CAD build for the part. Positions are in the model's coordinates, mm. A direction names the side the tool comes from. Give positions to 0.01 mm unless a question says otherwise; leave off trailing zeros. Write each loop counter-clockwise with the first axis right and the second up, starting at its lowest first coordinate (ties: lowest second). Pieces come first, ordered by that corner, then holes. Notation, with made-up numbers: M -36.75,-2.75 L 18.25,-2.75 A18 cw 18.25,19.25 Z; hole C 0,-1.5 d5. An arc over 180 degrees is marked long. One line per question, with ' | ' between items. Start each with the question number.
1. Pull direction X, two halves, no side cores. Call faces 1 (the face through (3.2, -3.2, 5.5)), 2 (the face through (1.75, 5, 3)), 3 (the face through (-7.493, 0.33, 2.712)), 4 (the face through (0, 6.15, 3)): released by +X, released by -X, zero draft, split by the parting line, or undercut.
2. Flat gauge pins, fed straight in: pin 1 (0.7 mm diameter, centred on y = 5, z = 2.5, fed in from -X); pin 2 (1.9 mm diameter, centred on y = 5.5, z = 1.5, fed in from +X); pin 3 (6 mm diameter, centred on x = -5.5, y = -2, fed in from -Z); pin 4 (2 mm diameter, centred on y = -2, z = 3.5, fed in from +X). Where does each tip first touch, or does it go through?
3. Cut at D-D, the plane x = 4.5. Write the cut outline in (y, z), then the cut area to 3 significant figures.
4. Wall check: L1, parallel to Y at x = 0, z = 3.4; L2, parallel to X at y = 4.5, z = 0.7; L3, parallel to X at y = -2, z = 4.5. Give the ranges that are in metal, low to high.
5. Cut at C-C, the plane y = 2. Write the cut outline in (x, z).
6. Cut at B-B, the plane z = 2.8. Write the cut outline in (x, y).
7. Cut at A-A, the plane x = 0. Write the cut outline in (y, z).
8. Which spindle directions (+Z, -Z, +X, -X, +Y, -Y) get a long thin tool onto all of the face, cutting with end or side? Do faces 5 (the face through (-1.75, 5, 3)), 6 (the face through (3.2, -3.2, 0)). Say none if no direction does.
```python
from build123d import *

# Parameters (mm, degrees)
SKIZZE1_R                       = 7.5
AUFSATZ_LINEAR_AUSTRAGEN1_DEPTH = 5.5


with BuildPart() as part:
    # Skizze1 → Aufsatz-Linear austragen1 (new body)
    with BuildSketch(Plane.XY):
        Circle(SKIZZE1_R)
        with BuildLine():
            ThreePointArc((4.15, 0), (-2.23159136, -3.498928407), (-1.75, 3.762977544))
            Line((-1.75, 3.762977544), (-1.75, 6.15))
            Line((-1.75, 6.15), (1.75, 6.15))
            Line((1.75, 6.15), (1.75, 3.762977544))
            ThreePointArc((1.75, 3.762977544), (3.498928407, 2.23159136), (4.15, 0))
        make_face(mode=Mode.SUBTRACT)
    extrude(amount=AUFSATZ_LINEAR_AUSTRAGEN1_DEPTH)


solid = part.part
```
Here are the results:
1) face 1: zero draft | face 2: undercut | face 3: split by the parting line | face 4: undercut
2) pin 1: x = -5.88 | pin 2: x = 5.96 | pin 3: z = 0 | pin 4: x = 7.43
3) outline: M -6,0 L 6,0 L 6,5.5 L -6,5.5 Z | area: 66.0 mm^2
4) L1: -7.5 to -4.15, 6.15 to 7.5 | L2: -6 to -1.75, 1.75 to 6 | L3: -7.23 to -3.64, 3.64 to 7.23
5) outline: M -7.23,0 L -3.64,0 L -3.64,5.5 L -7.23,5.5 Z; M 3.64,0 L 7.23,0 L 7.23,5.5 L 3.64,5.5 Z
6) outline: C 0,0 d15; hole M -1.75,3.76 A4.15 ccw long 1.75,3.76 L 1.75,6.15 L -1.75,6.15 Z
7) outline: M -7.5,0 L -4.15,0 L -4.15,5.5 L -7.5,5.5 Z; M 6.15,0 L 7.5,0 L 7.5,5.5 L 6.15,5.5 Z
8) face 5: +Z, -Z | face 6: -Z, +X, -X, +Y, -Y
